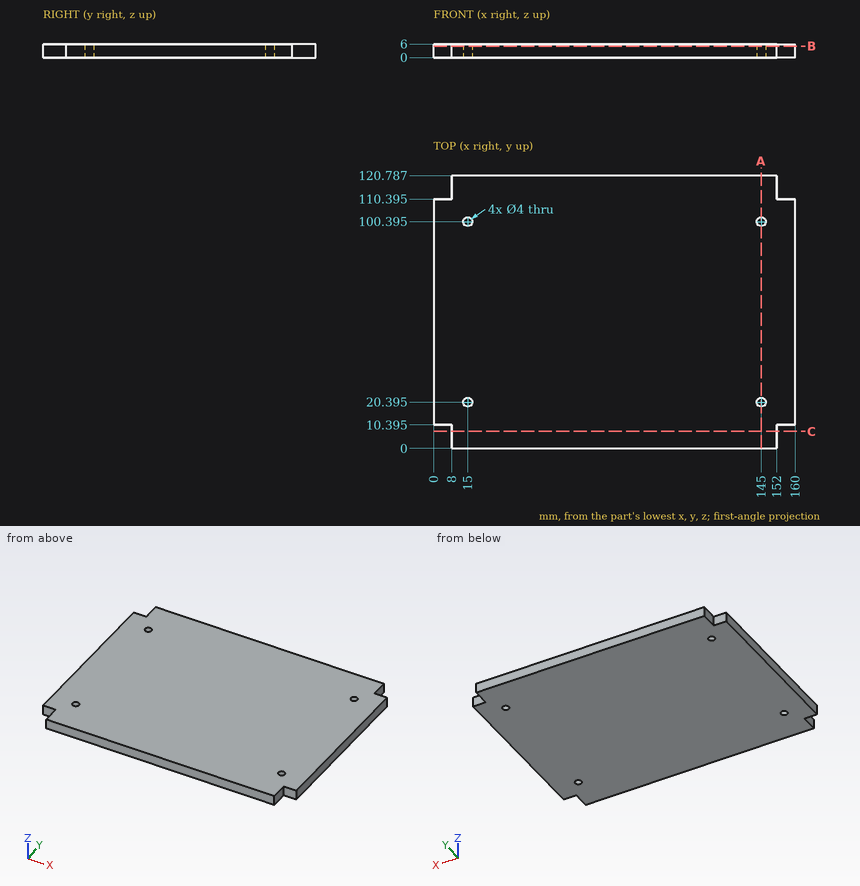
Geometry check sheet. Reference: drawing and pictorial views, mm from the part's lowest x, y, z. Coordinates: 2 decimals unless noted, no trailing zeros. Order: outer loops, then holes, each group sorted by start corner. A loop starts at its lowest first (then second) coordinate and runs counter-clockwise, first axis right, second up. Notation, with made-up numbers: (57, -5.5) -> (101, -5.5) arc R13 ccw to (101, 15.5) -> close; hole circle Ø4 at (-4, -33.75). An arc over 180 degrees is marked (long way). Write item = value, one per line. Start each with the question number.
1) Cross-section at B-B (z = 5.1). Enter the section's corners in (x, y) (1 decimal).
2) Cross-section at A-A (x = 145). Enter the section's corners in (y, z) (1 decimal), then the cut area to 3 significant figures.
3) Material ranges on L1, parallel to X at y = 100.5, z = 1.3; L2, parallel to Y at x = 145, z = 4.65 (1 decimal); L3, parallel to X at y = 9.5, z = 5.7, recorded low to high.
4) Cross-section at C-C (y = 7.5). Enter the section's corners in (x, z), then the cut area to 3 significant figures.
Ans:
q1.outline = (0, 10.4) -> (8, 10.4) -> (8, 0) -> (152, 0) -> (152, 10.4) -> (160, 10.4) -> (160, 110.4) -> (152, 110.4) -> (152, 120.8) -> (8, 120.8) -> (8, 110.4) -> (0, 110.4) -> close; hole circle Ø4 at (15, 20.4); hole circle Ø4 at (15, 100.4); hole circle Ø4 at (145, 20.4); hole circle Ø4 at (145, 100.4)
q2.outline = (0, 0) -> (18.4, 0) -> (18.4, 6) -> (0, 6) -> close; (22.4, 0) -> (98.4, 0) -> (98.4, 6) -> (22.4, 6) -> close; (102.4, 0) -> (120.8, 0) -> (120.8, 6) -> (102.4, 6) -> close
q2.area = 677 mm²
q3.L1 = 0 to 13, 17 to 143, 147 to 160
q3.L2 = 0 to 18.4, 22.4 to 98.4, 102.4 to 120.8
q3.L3 = 8 to 152
q4.outline = (8, 0) -> (152, 0) -> (152, 6) -> (8, 6) -> close
q4.area = 864 mm²
